Here's the drawing with two shaded views (mm, measured from the low corner). I have some questions. Give positions to 0.01 mm unless a question says otherwise; leave off trailing zeros. Write each loop counter-clockwise with the first axis right and the second up, starting at its lowest first coordinate (ties: lowest second). Pieces come first, ordered by that corner, then holes.
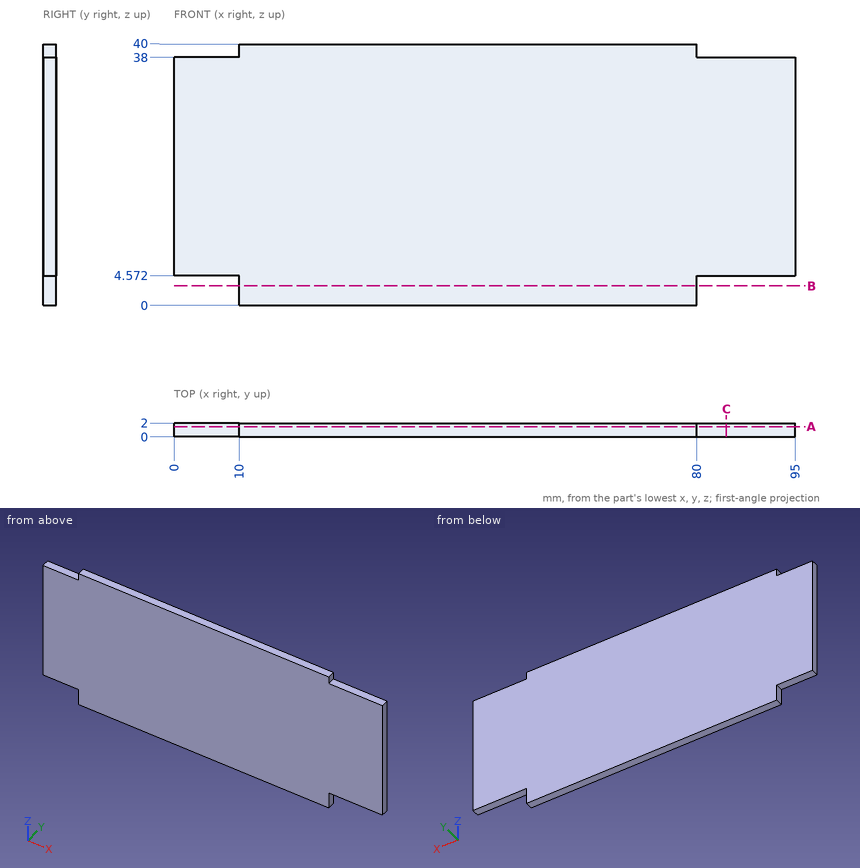
1) Suppose I cut it at C-C on x = 84.5. Write out the boundary of the cut face in (y, z).
Values follow:
outline: (0, 4.57) - (2, 4.57) - (2, 38) - (0, 38) - close
2) Please list where this line runs through material, in increasing order: L1, parallel to Z at x = 88.5, y = 1.1.
Values follow:
L1: z = 4.57 to 38
3) For pin 1 Ø1 at (x, y) = (4.5, 0.5) entering from +Z; pin 2 Ø0.6 at (y, z) = (0.5, 3.5) entering from +X; pin 3 Ø0.6 at (x, y) = (89, 0.5) entering from -Z, each with a flat end and sliding along its axis, tell me the tip position at first contact or that it passes through.
Values follow:
pin 1: stops at z = 38
pin 2: stops at x = 80
pin 3: stops at z = 4.57
4) Suppose I cut it at A-A on y = 1.5. Write out the boundary of the cut face in (x, z).
Values follow:
outline: (0, 4.57) - (10, 4.57) - (10, 0) - (80, 0) - (80, 4.57) - (95, 4.57) - (95, 38) - (80, 38) - (80, 40) - (10, 40) - (10, 38) - (0, 38) - close
5) Suppose I cut it at B-B on z = 3. Write out the boundary of the cut face in (x, y), plus the area to 3 significant figures.
Values follow:
outline: (10, 0) - (80, 0) - (80, 2) - (10, 2) - close
area: 140 mm2
